from build123d import *

# Parameters (mm, degrees)
ESBO_O1_W                = 23.7
ESBO_O1_H                = 18
RESSALTO_EXTRUS_O1_DEPTH = 1.1
ESBO_O2_W                = 8.7
ESBO_O2_H                = 6.3
RESSALTO_EXTRUS_O2_DEPTH = 3
FILETE1_R                = 1.5
ESBO_O3_R                = 1.420216844
ESBO_O3_W                = 1.821317375
ESBO_O3_H                = 1.611839717
ESBO_O3_W_2              = 1.876415965
ESBO_O3_W_3              = 1.749631103
ESBO_O3_H_2              = 1.434340909
CORTE_EXTRUS_O1_DEPTH    = 0.1
ESBO_O4_R                = 1
CORTE_EXTRUS_O2_DEPTH    = 31.711235729


with BuildPart() as part:
    # Esboço1 → Ressalto-extrusão1 (new body)
    with BuildSketch(Plane(origin=(0, 0, 0), x_dir=(1, 0, 0), z_dir=(0, 1, 0))):
        with Locations((11.85, 9)):
            Rectangle(ESBO_O1_W, ESBO_O1_H)
    extrude(amount=RESSALTO_EXTRUS_O1_DEPTH)

    # Esboço2 → Ressalto-extrusão2 (add)
    with BuildSketch(Plane(origin=(0, 1.1, 0), x_dir=(1, 0, 0), z_dir=(0, 1, 0))):
        with Locations((6.35, 16.15)):
            Rectangle(ESBO_O2_W, ESBO_O2_H)
    extrude(amount=RESSALTO_EXTRUS_O2_DEPTH)

    # Filete1
    filete1_edges = [part.edges().sort_by_distance(p)[0] for p in [
        (10.7, 1.1, -18.65),
        (2, 1.1, -18.65),
        (10.7, 4.1, -16.15),
        (2, 4.1, -16.15),
    ]]
    fillet(filete1_edges, radius=FILETE1_R - 0.0001)  # a hair under: the kernel refuses the full size

    # Esboço3 → Corte-extrusão1 (cut)
    with BuildSketch(Plane(origin=(0, 1.1, 0), x_dir=(1, 0, 0), z_dir=(0, 1, 0))):
        with Locations(Location((16.097292894, 10.816420735, 0), (0, 0, 270))):
            Circle(ESBO_O3_R)
        with Locations((0.910658688, 0.805919859)):
            Rectangle(ESBO_O3_W, ESBO_O3_H)
        with Locations((9.555193989, 0.805919859)):
            Rectangle(ESBO_O3_W_2, ESBO_O3_H)
        with Locations((13.143205597, 0.805919859)):
            Rectangle(ESBO_O3_W_3, ESBO_O3_H)
        with Locations((22.789341312, 0.717170455)):
            Rectangle(ESBO_O3_W, ESBO_O3_H_2)
    extrude(amount=-CORTE_EXTRUS_O1_DEPTH, mode=Mode.SUBTRACT)

    # Esboço4 → Corte-extrusão2 (cut, through all)
    with BuildSketch(Plane(origin=(0, 1.1, 0), x_dir=(1, 0, 0), z_dir=(0, 1, 0))):
        with Locations((0, 16)):
            Circle(ESBO_O4_R)
        with Locations((23.7, 16)):
            Circle(ESBO_O4_R)
    extrude(amount=-CORTE_EXTRUS_O2_DEPTH, mode=Mode.SUBTRACT)


solid = part.part
The model under review builds one solid part; all positions refer to its coordinate system, in mm. A direction names the side the tool comes from. Coordinates: 2 decimals unless noted, no trailing zeros. Loops run counter-clockwise (first coordinate to the right, second up) from the corner with the lowest first, then second, coordinate; pieces in that order, holes last. Notation, with made-up numbers: (-32.5, -1.5) -> (-15.5, -1.5) arc R11 ccw to (-15.5, 8.5) -> close; hole circle Ø6 at (-26.5, -19). An arc over 180 degrees is marked (long way). Use a Markdown table: item, result. Add a question column.
1. To check wall thickness, follow line 1 (Z direction, x = 4.25, y = 1.9); line 2 (X direction, y = 1.65, z = -14); line 3 (Z direction, x = 19.25, y = 0.65). State the ranges of each line that lie inside material, in increasing order.
2. Clearance check with flat-ended pins moving along their axes: pin 1 Ø0.9 at (x, z) = (16, -10.5) entering from +Y; pin 2 Ø0.9 at (x, y) = (5, 3) entering from +Z; pin 3 Ø1.3 at (x, z) = (9.5, -1) entering from +Y. State where each tip first meets the part, or that it passes through.
3. Add section C-C on y = 1.95. Write out the cut boundary in (x, z).
4. Add section D-D on z = -16. Write out the cut boundary in (x, y).
5. Draft analysis for pull direction Z (two halves, no side actions). For faces 6 (the face through (6, 3, -19.3)), 7 (the face through (22.7, 0.6, -16)), 8 (the face through (12, 0, -9)), state which applies: pulls with the +Z half, pulls with the -Z half, needs draft (parallel to the pull), parting line crosses it, or undercut.
6. Add section B-B on x = 5.25. Write out the cut boundary in (y, z).
7. Add section A-A on z = -13.5. Write out the cut boundary in (x, y).
8. Machinability: for faces 1 (the face through (6, 3, -13)), 2 (the face through (16, 1, -11)), 3 (the face through (13, 1, -1)), 4 (the face through (1, 1, -1)), 5 (the face through (2, 2, -15)), which of the approach directions +Z, -Z, +X, -X, +Y, -Y give a long, thin tool a straight path to every point of the face, cutting with its end or side? Answer none if there is none.
Returned:
| question | item | result |
|---|---|---|
| 1 | line 1 | z = -19.3 to -13 |
| 1 | line 2 | x = 2 to 10.7 |
| 1 | line 3 | z = -18 to 0 |
| 2 | pin 1 | stops at y = 1 |
| 2 | pin 2 | stops at z = -13 |
| 2 | pin 3 | stops at y = 1.1 |
| 3 | outline | (2, -18) -> (2.15, -18) -> (2.15, -19.3) -> (10.55, -19.3) -> (10.55, -18) -> (10.7, -18) -> (10.7, -13) -> (2, -13) -> close |
| 4 | outline | (1, 0) -> (22.7, 0) -> (22.7, 1.1) -> (10.7, 1.1) -> (10.7, 2.6) arc R1.5 ccw to (9.2, 4.1) -> (3.5, 4.1) arc R1.5 ccw to (2, 2.6) -> (2, 1.1) -> (1, 1.1) -> close |
| 5 | face 6 | pulls with the -Z half |
| 5 | face 7 | undercut |
| 5 | face 8 | needs draft |
| 6 | outline | (0, -18) -> (1.1, -18) -> (1.1, -19.3) -> (4.1, -19.3) -> (4.1, -13) -> (1.1, -13) -> (1.1, 0) -> (0, 0) -> close |
| 7 | outline | (0, 0) -> (23.7, 0) -> (23.7, 1.1) -> (10.7, 1.1) -> (10.7, 2.6) arc R1.5 ccw to (9.2, 4.1) -> (3.5, 4.1) arc R1.5 ccw to (2, 2.6) -> (2, 1.1) -> (0, 1.1) -> close |
| 8 | face 1 | +Z, +X, -X, +Y |
| 8 | face 2 | +Y |
| 8 | face 3 | +Z, +Y |
| 8 | face 4 | +Z, -X, +Y |
| 8 | face 5 | +Z, -Z, -X, +Y |
